The listing builds one solid part. Answer for the finished solid, in the listing's coordinates (mm). Give positions to 0.01 mm unless a question says otherwise; leave off trailing zeros. Use a Markdown table: item, result. Add a question column.
1) Find section A-A, the plane x = 127.5. State how many separate pieces and enclosed holes the cut face has, plus the area to 3 significant figures.
2) Straight lines are drawn through the part: line 1 (Y direction, x = 196, z = 10); line 2 (Y direction, x = 236.5, z = -5); line 3 (Z direction, x = 375, y = 2). For each, find the intervals that lie inside material, in ascending order.
3) Flat-ended cylindrical pins translate along their axes: pin 1 (1.5 mm diameter, centred on x = 184, z = 11.5, fed in from -Y); pin 2 (3 mm diameter, centred on x = 244, z = -11, fed in from +Y); pin 3 (3 mm diameter, centred on x = 73, z = -12, fed in from -Y); pin 4 (3 mm diameter, centred on x = 131.5, y = 0, fed in from -Z). Find the tip coordinate at first contact, or state that the pin passes through.
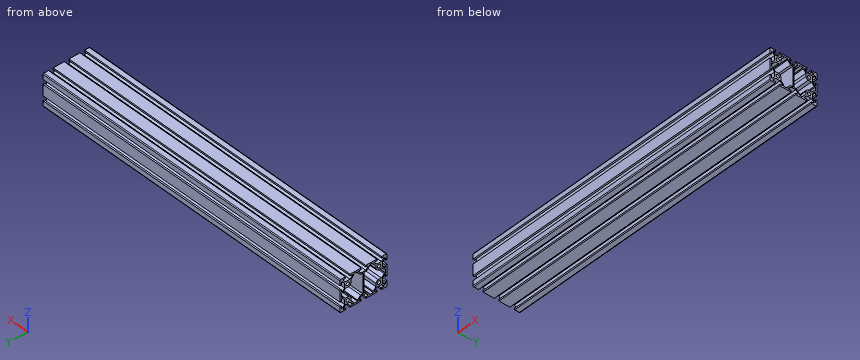
from build123d import *

# Parameters (mm, degrees)
SKETCH1_R           = 2.1
BOSS_EXTRUDE1_DEPTH = 420


with BuildPart() as part:
    # Sketch1 → Boss-Extrude1 (new body)
    with BuildSketch(Plane(origin=(0, 0, 0), x_dir=(0, 0, -1), z_dir=(1, 0, 0))):
        with BuildLine():
            Line((-20, 29), (-20, 23))
            Line((-20, 23), (-18, 23))
            Line((-18, 23), (-18, 26))
            Line((-18, 26), (-17.060660172, 26))
            Line((-17.060660172, 26), (-14, 22.939339828))
            Line((-14, 22.939339828), (-14, 17.060660172))
            Line((-14, 17.060660172), (-17.060660172, 14))
            Line((-17.060660172, 14), (-18, 14))
            Line((-18, 14), (-18, 17))
            Line((-18, 17), (-20, 17))
            Line((-20, 17), (-20, 3))
            Line((-20, 3), (-18, 3))
            Line((-18, 3), (-18, 6))
            Line((-18, 6), (-17.060660172, 6))
            Line((-17.060660172, 6), (-14, 2.939339828))
            Line((-14, 2.939339828), (-14, -2.939339828))
            Line((-14, -2.939339828), (-17.060660172, -6))
            Line((-17.060660172, -6), (-18, -6))
            Line((-18, -6), (-18, -3))
            Line((-18, -3), (-20, -3))
            Line((-20, -3), (-20, -17))
            Line((-20, -17), (-18, -17))
            Line((-18, -17), (-18, -14))
            Line((-18, -14), (-17.060660172, -14))
            Line((-17.060660172, -14), (-14, -17.060660172))
            Line((-14, -17.060660172), (-14, -22.939339828))
            Line((-14, -22.939339828), (-17.060660172, -26))
            Line((-17.060660172, -26), (-18, -26))
            Line((-18, -26), (-18, -23))
            Line((-18, -23), (-20, -23))
            Line((-20, -23), (-20, -29))
            ThreePointArc((-20, -29), (-19.707106781, -29.707106781), (-19, -30))
            Line((-19, -30), (-13, -30))
            Line((-13, -30), (-13, -28))
            Line((-13, -28), (-16, -28))
            Line((-16, -28), (-16, -27.060660172))
            Line((-16, -27.060660172), (-12.939339828, -24))
            Line((-12.939339828, -24), (-7.060660172, -24))
            Line((-7.060660172, -24), (-4, -27.060660172))
            Line((-4, -27.060660172), (-4, -28))
            Line((-4, -28), (-7, -28))
            Line((-7, -28), (-7, -30))
            Line((-7, -30), (7, -30))
            Line((7, -30), (7, -28))
            Line((7, -28), (4, -28))
            Line((4, -28), (4, -27.060660172))
            Line((4, -27.060660172), (7.060660172, -24))
            Line((7.060660172, -24), (12.939339828, -24))
            Line((12.939339828, -24), (16, -27.060660172))
            Line((16, -27.060660172), (16, -28))
            Line((16, -28), (13, -28))
            Line((13, -28), (13, -30))
            Line((13, -30), (19, -30))
            ThreePointArc((19, -30), (19.707106781, -29.707106781), (20, -29))
            Line((20, -29), (20, -23))
            Line((20, -23), (18, -23))
            Line((18, -23), (18, -26))
            Line((18, -26), (17.060660172, -26))
            Line((17.060660172, -26), (14, -22.939339828))
            Line((14, -22.939339828), (14, -17.060660172))
            Line((14, -17.060660172), (17.060660172, -14))
            Line((17.060660172, -14), (18, -14))
            Line((18, -14), (18, -17))
            Line((18, -17), (20, -17))
            Line((20, -17), (20, -3))
            Line((20, -3), (18, -3))
            Line((18, -3), (18, -6))
            Line((18, -6), (17.060660172, -6))
            Line((17.060660172, -6), (14, -2.939339828))
            Line((14, -2.939339828), (14, 2.939339828))
            Line((14, 2.939339828), (17.060660172, 6))
            Line((17.060660172, 6), (18, 6))
            Line((18, 6), (18, 3))
            Line((18, 3), (20, 3))
            Line((20, 3), (20, 17))
            Line((20, 17), (18, 17))
            Line((18, 17), (18, 14))
            Line((18, 14), (17.060660172, 14))
            Line((17.060660172, 14), (14, 17.060660172))
            Line((14, 17.060660172), (14, 22.939339828))
            Line((14, 22.939339828), (17.060660172, 26))
            Line((17.060660172, 26), (18, 26))
            Line((18, 26), (18, 23))
            Line((18, 23), (20, 23))
            Line((20, 23), (20, 29))
            ThreePointArc((20, 29), (19.707106781, 29.707106781), (19, 30))
            Line((19, 30), (13, 30))
            Line((13, 30), (13, 28))
            Line((13, 28), (16, 28))
            Line((16, 28), (16, 27.060660172))
            Line((16, 27.060660172), (12.939339828, 24))
            Line((12.939339828, 24), (7.060660172, 24))
            Line((7.060660172, 24), (4, 27.060660172))
            Line((4, 27.060660172), (4, 28))
            Line((4, 28), (7, 28))
            Line((7, 28), (7, 30))
            Line((7, 30), (-7, 30))
            Line((-7, 30), (-7, 28))
            Line((-7, 28), (-4, 28))
            Line((-4, 28), (-4, 27.060660172))
            Line((-4, 27.060660172), (-7.060660172, 24))
            Line((-7.060660172, 24), (-12.939339828, 24))
            Line((-12.939339828, 24), (-16, 27.060660172))
            Line((-16, 27.060660172), (-16, 28))
            Line((-16, 28), (-13, 28))
            Line((-13, 28), (-13, 30))
            Line((-13, 30), (-19, 30))
            ThreePointArc((-19, 30), (-19.707106781, 29.707106781), (-20, 29))
        make_face()
        with Locations((-10, 20)):
            Circle(SKETCH1_R, mode=Mode.SUBTRACT)
        with Locations((10, 20)):
            Circle(SKETCH1_R, mode=Mode.SUBTRACT)
        with Locations((10, -20)):
            Circle(SKETCH1_R, mode=Mode.SUBTRACT)
        with Locations((-10, -20)):
            Circle(SKETCH1_R, mode=Mode.SUBTRACT)
        with BuildLine():
            Line((-16.439339828, 12.5), (-18, 12.5))
            Line((-18, 12.5), (-18, 7.5))
            Line((-18, 7.5), (-16.439339828, 7.5))
            Line((-16.439339828, 7.5), (-12.5, 3.560660172))
            Line((-12.5, 3.560660172), (-12.5, 0.75))
            Line((-12.5, 0.75), (12.5, 0.75))
            Line((12.5, 0.75), (12.5, 3.560660172))
            Line((12.5, 3.560660172), (16.439339828, 7.5))
            Line((16.439339828, 7.5), (18, 7.5))
            Line((18, 7.5), (18, 12.5))
            Line((18, 12.5), (16.439339828, 12.5))
            Line((16.439339828, 12.5), (12.939339828, 16))
            Line((12.939339828, 16), (9, 16))
            ThreePointArc((9, 16), (6.878679656, 16.878679656), (6, 19))
            Line((6, 19), (6, 22.939339828))
            Line((6, 22.939339828), (2.5, 26.439339828))
            Line((2.5, 26.439339828), (2.5, 28))
            Line((2.5, 28), (-2.5, 28))
            Line((-2.5, 28), (-2.5, 26.439339828))
            Line((-2.5, 26.439339828), (-6, 22.939339828))
            Line((-6, 22.939339828), (-6, 19))
            ThreePointArc((-6, 19), (-6.878679656, 16.878679656), (-9, 16))
            Line((-9, 16), (-12.939339828, 16))
            Line((-12.939339828, 16), (-16.439339828, 12.5))
        make_face(mode=Mode.SUBTRACT)
        with BuildLine():
            Line((-18, -7.5), (-18, -12.5))
            Line((-18, -12.5), (-16.439339828, -12.5))
            Line((-16.439339828, -12.5), (-12.939339828, -16))
            Line((-12.939339828, -16), (-9, -16))
            ThreePointArc((-9, -16), (-6.878679656, -16.878679656), (-6, -19))
            Line((-6, -19), (-6, -22.939339828))
            Line((-6, -22.939339828), (-2.5, -26.439339828))
            Line((-2.5, -26.439339828), (-2.5, -28))
            Line((-2.5, -28), (2.5, -28))
            Line((2.5, -28), (2.5, -26.439339828))
            Line((2.5, -26.439339828), (6, -22.939339828))
            Line((6, -22.939339828), (6, -19))
            ThreePointArc((6, -19), (6.878679656, -16.878679656), (9, -16))
            Line((9, -16), (12.939339828, -16))
            Line((12.939339828, -16), (16.439339828, -12.5))
            Line((16.439339828, -12.5), (18, -12.5))
            Line((18, -12.5), (18, -7.5))
            Line((18, -7.5), (16.439339828, -7.5))
            Line((16.439339828, -7.5), (12.5, -3.560660172))
            Line((12.5, -3.560660172), (12.5, -0.75))
            Line((12.5, -0.75), (-12.5, -0.75))
            Line((-12.5, -0.75), (-12.5, -3.560660172))
            Line((-12.5, -3.560660172), (-16.439339828, -7.5))
            Line((-16.439339828, -7.5), (-18, -7.5))
        make_face(mode=Mode.SUBTRACT)
    extrude(amount=BOSS_EXTRUDE1_DEPTH)


solid = part.part
The answers:
| question | item | result |
|---|---|---|
| 1 | separate pieces | 1 |
| 1 | enclosed holes | 6 |
| 1 | area | 654 mm2 |
| 2 | line 1 | -24 to -22.1, -17.9 to -16, -0.75 to 0.75, 16 to 17.9, 22.1 to 24 |
| 2 | line 2 | -30 to -28, -26.06 to -23.94, -0.75 to 0.75, 23.94 to 26.06, 28 to 30 |
| 2 | line 3 | -14 to -12.5, 12.5 to 14 |
| 3 | pin 1 | y = -24 |
| 3 | pin 2 | y = 24 |
| 3 | pin 3 | y = -30 |
| 3 | pin 4 | z = -14 |
